from build123d import *


with BuildPart() as part:
    # Pushrod Sketch → Pushrod (revolve)
    with BuildSketch(Plane.XY, mode=Mode.PRIVATE) as pushrod_sk:
        Polygon((-4, 0), (-3.894878566, 0.910999976), (-3.585039521, 1.774117141), (-3.086768229, 2.543985436), (-2.426254185, 3.180140033), (-1.638214481, 3.649144189), (-0.76406905, 3.92634671), (0.150236399, 3.997177632), (1.056645315, 3.857914032), (1.907516195, 3.515875704), (2.658126657, 2.989040428), (3.269024075, 2.305099043), (3.708099244, 1.5), (41.272452109, 1.5), (41.711527278, 2.305099043), (42.322424696, 2.989040428), (43.073035158, 3.515875704), (43.923906038, 3.857914032), (44.830314954, 3.997177632), (45.744620403, 3.92634671), (46.618765834, 3.649144189), (47.406805538, 3.180140033), (48.067319582, 2.543985436), (48.565590874, 1.774117141), (48.875429919, 0.910999976), (48.980551353, 0), align=None)
    revolve(pushrod_sk.sketch.rotate(Axis((-1000, 0, 0), (1, 0, 0)), 90), axis=Axis((-1000, 0, 0), (1, 0, 0)))


solid = part.part
Build history of the part. All positions in model axes, mm. Round coordinates to 2 decimals unless told otherwise and drop trailing zeros. Loops run counter-clockwise (first coordinate to the right, second up) from the corner with the lowest first, then second, coordinate; pieces in that order, holes last. Notation, with made-up numbers: (-34.5, 22) -> (-19.5, 22) arc R6 cw to (-19.5, 31) -> close; hole circle Ø6 at (71, 56). An arc over 180 degrees is marked (long way). Answer in a Markdown table with one row per item.
Item 1: Saw through at A-A (x = 7). Write the cut outline in (y, z), and give its area (3 significant figures).
Answers below:
| item | result |
|---|---|
| outline | circle Ø3 at (0, 0) |
| area | 7.07 mm² |
Item 2: Drill centre lines: L1, parallel to X at y = -2, z = 3; L2, parallel to X at y = 3.25, z = 1.5; L3, parallel to Y at x = 38, z = -0.5. Where is each one in solid material? Low to high. Write a range as [from, to].
Answers below:
| item | result |
|---|---|
| L1 | x = [-1.71, 1.68], [43.3, 46.69] |
| L2 | x = [-1.76, 1.75], [43.23, 46.74] |
| L3 | y = [-1.41, 1.41] |
Item 3: Pin check, flat tips, straight feed: pin 1 (2 mm diameter, centred on x = 41.5, z = 0.5, fed in from +Y); pin 2 (2 mm diameter, centred on x = 3.5, z = -1, fed in from -Y); pin 3 (4 mm diameter, centred on x = 32.5, z = 0.5, fed in from -Y). Stop position of each tip, or through.
Answers below:
| item | result |
|---|---|
| pin 1 | stops at y = 3.09 |
| pin 2 | stops at y = -2.99 |
| pin 3 | stops at y = -1.5 |
